The model under review builds one solid part; all positions refer to its coordinate system, in mm. Face numbers are marked on the shaded views. A direction names the side the tool comes from. Coordinates: 2 decimals unless noted, no trailing zeros. Write each loop counter-clockwise with the first axis right and the second up, starting at its lowest first coordinate (ties: lowest second). Pieces come first, ordered by that corner, then holes. Notation, with made-up numbers: M 83.5,13 L 125.5,13 A17 cw 125.5,23 Z; hole C 76.5,62.5 d8. An arc over 180 degrees is marked long. Answer as a JSON object with one key per item and string values.
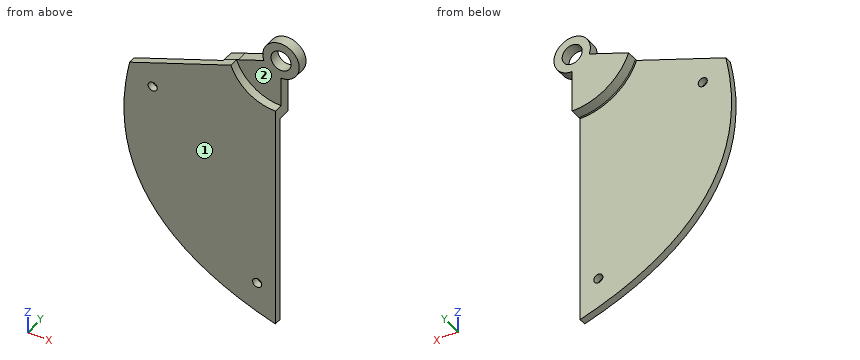
Autodesk Inventor part; units mm, degrees
ref_plane "YZ Plane" through (0, 0, 0) normal (1, 0, 0) x (0, 1, 0)
ref_plane "XZ Plane" through (0, 0, 0) normal (0, 1, 0) x (-1, 0, 0)
ref_plane "XY Plane" through (0, 0, 0) normal (0, 0, 1) x (1, 0, 0)
sketch "Sketch1" plane through (0, 0, 0) normal (0, 1, 0) x (-1, 0, 0)
  circle A0 centre (0, 0) radius 12.5
  line L0 (11.7462, -4.2753) -> (40, -14.5588)
  line L1 (0, 0) -> (41.7481, 0) construction
  line L2 (0, 0) -> (11.7462, -4.2753) construction
  line L3 (0, 0) -> (0, -75)
  line L4 (0, -75) -> (27.0598, -66.8927) construction
  line L5 (27.0598, -66.8927) -> (47.507, -49.1207) construction
  line L6 (47.507, -49.1207) -> (40, -14.5588) construction
  spline S0 degree 3 poles (0, -75) (27.0598, -66.8927) (47.507, -49.1207) (40, -14.5588) knots 1 1 1 1 2 2 2 2
  point P0 (0, -12.5)
  dimension "d0" = 25
  dimension "d1" = 40
  dimension "d3" = 20
  dimension "d4" = 75
extrude "Extrusion1" add sketch "Sketch1" along normal blind 2
sketch "Sketch2" plane through (0, 0, 0) normal (0, -1, 0) x (1, 0, 0)
  circle A0 centre (0, 0) radius 2.5
  dimension "d7" = 5
extrude "Extrusion2" add sketch "Sketch2" along normal blind 4
sketch "Sketch3" plane through (0, 0, 0) normal (0, -1, 0) x (1, 0, 0)
  arc A0 (11.7462, -4.2753) -> (0, -12.5) centre (0, 0) ccw
  arc A1 (0, -12.5) -> (-11.7462, -4.2753) centre (0, 0) ccw
extrude "Extrusion3" cut sketch "Sketch3" against normal mid plane 10
sketch "Sketch4" plane through (0, 2, 0) normal (0, 1, 0) x (1, 0, 0)
  circle A0 centre (0, 0) radius 16.5
  arc A1 (0, 12.5) -> (-11.7462, 4.2753) centre (0, 0) ccw
  circle A2 centre (0, 0) radius 4.8598
  line L0 (-40, 14.5588) -> (-11.7462, 4.2753)
  line L1 (0, 12.5) -> (0, 75)
  point P0 (0, 16.5)
  point P1 (-15.5049, 5.6433)
  dimension "d12" = 4
  dimension "d13" = 9.7195
extrude "Extrusion4" add sketch "Sketch4" along normal blind 0.5 contours L1 A1 L0 A0 picked at (-4.9207, 14.2357)
sketch "Sketch5" plane through (0, 2.5, 0) normal (0, 1, 0) x (1, 0, 0)
  circle A0 centre (0, 0) radius 5
  arc A1 (0, 12.5) -> (-11.7462, 4.2753) centre (0, 0) ccw
  line L0 (0, 5) -> (0, 12.5)
  line L1 (-11.7462, 4.2753) -> (-4.6985, 1.7101)
  line L2 (-15.5049, 5.6433) -> (-11.7462, 4.2753)
  line L3 (0, 12.5) -> (0, 16.5)
  arc A2 (0, 16.5) -> (-15.5049, 5.6433) centre (0, 0) ccw
  circle A3 centre (0, 0) radius 2.75
  dimension "d16" = 10
  dimension "d17" = 5.5
extrude "Extrusion5" add sketch "Sketch5" along normal blind 3
sketch "Sketch6" plane through (0, 0, 0) normal (0, -1, 0) x (1, 0, 0)
  arc A0 (-11.7462, -4.2753) -> (0, -12.5) centre (0, 0) ccw
  line L0 (0, -12.5) -> (0, -75)
  line L1 (-40, -14.5588) -> (-11.7462, -4.2753)
  circle A1 centre (0, 0) radius 2.75
  circle A2 centre (0, 0) radius 13
  point P0 (-12.216, -4.4463)
  point P1 (0, -13)
  dimension "d20" = 0.5
extrude "Extrusion6" cut sketch "Sketch6" against normal up to surface (2.5 mm away) contours A0 L0 A2 L1 picked at (-1.0483, -12.7046)
sketch "Sketch7" plane through (0, 0, 0) normal (0, -1, 0) x (1, 0, 0)
  circle A0 centre (-5, -65) radius 1.25
  circle A1 centre (-33.6672, -19.171) radius 1.25
  line L0 (-40, -14.5588) -> (-12.216, -4.4463)
  point P0 (0, 0)
  dimension "d23" = 6.5
  dimension "d24" = 19.171
  dimension "d25" = 2.5
  dimension "d26" = 65
  dimension "d27" = 5
extrude "Extrusion7" cut sketch "Sketch7" against normal up to surface (2 mm away)
equation "\"d28\" = d25"
properties part number "clamshell half-2" material "ABS Plastic"
(1) Add section A-A on z = 0. Give the boundary of the cut face in (x, y).
Results list:
{"outline": "M -5,2.5 L -2.75,2.5 L -2.75,5.5 L -5,5.5 Z; M 2.75,2.5 L 5,2.5 L 5,5.5 L 2.75,5.5 Z"}
(2) For the marked faces 1 and 2, list the 3-axis set-ups (+Z, -Z, +X, -X, +Y, -Y) from which the entire face can be reached by the end or side of a thin tool; tool diameter is ignored.
Results list:
{"face 1": "+Z, -Z, +X, -X, -Y", "face 2": "+Z, +X, -Y"}
(3) For pin 1 Ø4.5 at (x, z) = (0, 0) entering from +Y; pin 2 Ø3 at (x, y) = (-36, 1.5) entering from -Z; pin 3 Ø3 at (x, y) = (-30, 2.5) entering from -Z; pin 4 Ø1.5 at (x, z) = (-18.5, -17.5) entering from +Y, all flat-tipped, find the tip position at first contact; note any pin that passes through.
Results list:
{"pin 1": "through", "pin 2": "z = -52.58", "pin 3": "z = -59.56", "pin 4": "y = 2"}
(4) Wall thickness on line 1 along X through (y, z) = (4.8, 0); line 2 along Y through (x, z) = (-32.5, -36.5); line 3 along Z through (x, y) = (-2, 2.75): over which ranges is each line inside the solid? List them lowest first. Write a range as from..to.
Results list:
{"line 1": "-5..-2.75, 2.75..5", "line 2": "0..2", "line 3": "-16.38..-1.89, 1.89..4.58"}
